Autodesk Inventor part; units mm, degrees
ref_plane "CP_XY" through (0, 0, 0) normal (0, 1, 0) x (1, 0, 0)
ref_plane "CP_YZ" through (0, 0, 0) normal (1, 0, 0) x (0, 0, -1)
ref_plane "CP_ZX" through (0, 0, 0) normal (0, 0, -1) x (0, 1, 0)
sketch "Sketch_1" plane through (0, 0, 0) normal (1, 0, 0) x (0, 1, 0)
  line L0 (6.8, 43.4562) -> (3.8228, 41.7889)
  arc A0 (3.8228, 41.7889) -> (2.8, 40.0439) centre (4.8, 40.0439) ccw
  line L1 (2.8, 40.0439) -> (2.8, -40.0439)
  arc A1 (2.8, -40.0439) -> (3.8228, -41.7889) centre (4.8, -40.0439) ccw
  line L2 (3.8228, -41.7889) -> (5.3114, -42.6226)
  arc A2 (5.3114, -42.6226) -> (6.8, -41.7501) centre (5.8, -41.7501) ccw
  line L3 (6.8, -41.7501) -> (6.8, 43.4562)
extrude "Extrusion1" add sketch "Sketch_1" along normal mid plane 22.5
sketch "Sketch_4" plane through (0, 0, 0) normal (1, 0, 0) x (0, 1, 0)
  line L0 (6.78, 48.4) -> (-1, 48.4)
  line L1 (-1, 48.4) -> (-1, -48.4)
  line L2 (-1, -48.4) -> (6.78, -48.4)
  line L3 (6.78, -48.4) -> (7.1588, -48.2985)
  arc A0 (7.1588, -48.2985) -> (7.9, -47.3326) centre (6.9, -47.3326) ccw
  line L4 (7.9, -47.3326) -> (7.9, -45.0762)
  arc A1 (7.9, -45.0762) -> (7.3886, -44.2037) centre (6.9, -45.0762) ccw
  line L5 (7.3886, -44.2037) -> (5.4, -43.09)
  line L6 (5.4, -43.09) -> (5.4, 43.09)
  line L7 (5.4, 43.09) -> (7.3886, 44.2037)
  arc A2 (7.3886, 44.2037) -> (7.9, 45.0762) centre (6.9, 45.0762) ccw
  line L8 (7.9, 45.0762) -> (7.9, 47.3326)
  arc A3 (7.9, 47.3326) -> (7.1588, 48.2985) centre (6.9, 47.3326) ccw
  line L9 (7.1588, 48.2985) -> (6.78, 48.4)
extrude "Extrusion2" cut sketch "Sketch_4" along normal mid plane 20
sketch "Sketch_10" plane through (5.5, 0, 0) normal (1, 0, 0) x (0, 0, -1)
  line L0 (-43.5, 6.7302) -> (-42.755, 5.4)
  line L1 (-42.755, 5.4) -> (-42.2975, 5.4)
  line L2 (-42.2975, 5.4) -> (-41.9848, 7.1736)
  arc A0 (-40.0152, 7.1736) -> (-41.9848, 7.1736) centre (-41, 7) ccw
  line L3 (-40.0152, 7.1736) -> (-39.7025, 5.4)
  line L4 (-39.7025, 5.4) -> (-37.8117, 5.4)
  line L5 (-37.8117, 5.4) -> (-39.255, 7.9772)
  arc A1 (-39.255, 7.9772) -> (-42.7116, 8.0346) centre (-41, 7) ccw
  line L6 (-42.7116, 8.0346) -> (-43.5, 6.7302)
extrude "Extrusion3" add sketch "Sketch_10" against normal blind 1.4
sketch "Sketch_2" plane through (-5.5, 0, 0) normal (1, 0, 0) x (0, 0, -1)
  line L0 (-43.5, 6.7302) -> (-42.755, 5.4)
  line L1 (-42.755, 5.4) -> (-42.2975, 5.4)
  line L2 (-42.2975, 5.4) -> (-41.9848, 7.1736)
  arc A0 (-40.0152, 7.1736) -> (-41.9848, 7.1736) centre (-41, 7) ccw
  line L3 (-40.0152, 7.1736) -> (-39.7025, 5.4)
  line L4 (-39.7025, 5.4) -> (-37.8117, 5.4)
  line L5 (-37.8117, 5.4) -> (-39.255, 7.9772)
  arc A1 (-39.255, 7.9772) -> (-42.7116, 8.0346) centre (-41, 7) ccw
  line L6 (-42.7116, 8.0346) -> (-43.5, 6.7302)
extrude "Extrusion4" add sketch "Sketch_2" along normal blind 1.4
sketch "Sketch_3" plane through (0, 0, 0) normal (1, 0, 0) x (0, 1, 0)
  line L0 (7.3, 45) -> (2.8, 45)
  line L1 (2.8, 45) -> (2.8, 41.2161)
  line L2 (2.8, 41.2161) -> (6.7545, 43.4307)
  arc A0 (6.8522, 43.4562) -> (6.7545, 43.4307) centre (6.8522, 43.2562) ccw
  line L3 (6.8522, 43.4562) -> (7.3, 43.4562)
  line L4 (7.3, 43.4562) -> (7.3, 45)
extrude "Extrusion5" cut sketch "Sketch_3" along normal mid plane 24
sketch "Sketch_5" plane through (0, 6.8, 0) normal (0, 1, 0) x (1, 0, 0)
  line L0 (-4.1, -38.44) -> (-4.1, -47)
  line L1 (-4.1, -47) -> (4.1, -47)
  line L2 (4.1, -47) -> (4.1, -38.44)
  line L3 (4.1, -38.44) -> (1.9, -38.44)
  line L4 (1.9, -38.44) -> (1.9, -45)
  line L5 (1.9, -45) -> (-1.9, -45)
  line L6 (-1.9, -45) -> (-1.9, -38.44)
  line L7 (-1.9, -38.44) -> (-4.1, -38.44)
extrude "Extrusion6" cut sketch "Sketch_5" against normal blind 1.5
sketch "Sketch_6" plane through (5.5, 0, 0) normal (1, 0, 0) x (0, 0, -1)
  line L0 (-42.2975, 5.4) -> (-39.7025, 5.4)
  line L1 (-39.7025, 5.4) -> (-40.0152, 7.1736)
  arc A0 (-40.0152, 7.1736) -> (-41.9848, 7.1736) centre (-41, 7) ccw
  line L2 (-41.9848, 7.1736) -> (-42.2975, 5.4)
extrude "Extrusion7" cut sketch "Sketch_6" against normal blind 1.5
sketch "Sketch_7" plane through (-5.5, 0, 0) normal (1, 0, 0) x (0, 0, -1)
  line L0 (-42.2975, 5.4) -> (-39.7025, 5.4)
  line L1 (-39.7025, 5.4) -> (-40.0152, 7.1736)
  arc A0 (-40.0152, 7.1736) -> (-41.9848, 7.1736) centre (-41, 7) ccw
  line L2 (-41.9848, 7.1736) -> (-42.2975, 5.4)
extrude "Extrusion8" cut sketch "Sketch_7" along normal blind 1.5
sketch "Sketch_8" plane through (0, 6.8, 0) normal (0, 1, 0) x (1, 0, 0)
  line L0 (-9.1, 46) -> (-9.1, 38.25)
  arc A0 (-9.1, 38.25) -> (-8.5, 37.65) centre (-8.5, 38.25) ccw
  line L1 (-8.5, 37.65) -> (-7.331, 37.65)
  arc A1 (-7.331, 37.65) -> (-7.0913, 37.829) centre (-7.331, 37.9) ccw
  line L2 (-7.0913, 37.829) -> (-6.7103, 39.1152)
  arc A2 (-6.7103, 39.1152) -> (-6.7, 39.1862) centre (-6.95, 39.1862) ccw
  line L3 (-6.7, 39.1862) -> (-6.7, 44)
  line L4 (-6.7, 44) -> (6.7, 44)
  line L5 (6.7, 44) -> (6.7, 39.1862)
  arc A3 (6.7, 39.1862) -> (6.7103, 39.1152) centre (6.95, 39.1862) ccw
  line L6 (6.7103, 39.1152) -> (7.0913, 37.829)
  arc A4 (7.0913, 37.829) -> (7.331, 37.65) centre (7.331, 37.9) ccw
  line L7 (7.331, 37.65) -> (8.5, 37.65)
  arc A5 (8.5, 37.65) -> (9.1, 38.25) centre (8.5, 38.25) ccw
  line L8 (9.1, 38.25) -> (9.1, 46)
  line L9 (9.1, 46) -> (-9.1, 46)
extrude "Extrusion9" cut sketch "Sketch_8" against normal blind 1.5
sketch "Sketch_11" plane through (0, 6.8, 0) normal (0, 1, 0) x (1, 0, 0)
  line L0 (-6.95, 28.75) -> (6.95, 28.75)
  line L1 (6.95, 28.75) -> (6.95, 37.05)
  line L2 (6.95, 37.05) -> (-6.95, 37.05)
  line L3 (-6.95, 37.05) -> (-6.95, 28.75)
extrude "Extrusion10" cut sketch "Sketch_11" against normal blind 0.5
sketch "Sketch_13" plane through (0, 6.8, 0) normal (0, 1, 0) x (1, 0, 0)
  circle A0 centre (-5, 32.9) radius 0.6
extrude "Extrusion11" cut sketch "Sketch_13" against normal blind 1.5
sketch "Sketch_14" plane through (0, 6.8, 0) normal (0, 1, 0) x (1, 0, 0)
  circle A0 centre (5, 32.9) radius 0.6
extrude "Extrusion12" cut sketch "Sketch_14" against normal blind 1.5
ref_plane "CP_XY" through (0, 0, 0) normal (0, 1, 0) x (1, 0, 0)
ref_plane "CP_YZ" through (0, 0, 0) normal (1, 0, 0) x (0, 0, -1)
ref_plane "CP_ZX" through (0, 0, 0) normal (0, 0, -1) x (0, 1, 0)
ref_plane "mitFront_XY" through (0, 7, 41) normal (1, 0, 0) x (0, 0, -1)
ref_plane "mitFront_YZ" through (0, 7, 41) normal (0, 0, -1) x (0, 1, 0)
ref_plane "mitFront_ZX" through (0, 7, 41) normal (0, 1, 0) x (1, 0, 0)
ref_plane "mitMark_XY" through (0, 6.3, -32.9) normal (0, -1, 0) x (1, 0, 0)
ref_plane "mitMark_YZ" through (0, 6.3, -32.9) normal (1, 0, 0) x (0, 0, 1)
ref_plane "mitMark_ZX" through (0, 6.3, -32.9) normal (0, 0, 1) x (0, -1, 0)
properties part number "CH20M22 C BK 2418670000"
The listing builds one solid part. Answer for the finished solid, in the listing's coordinates (mm). A direction names the side the tool comes from. Coordinates: 2 decimals unless noted, no trailing zeros. Write each loop counter-clockwise with the first axis right and the second up, starting at its lowest first coordinate (ties: lowest second). Pieces come first, ordered by that corner, then holes. Notation, with made-up numbers: M 39.25,-13 L 94.25,-13 A23 cw 94.25,0 Z; hole C -29,51.5 d3. An arc over 180 degrees is marked long. Put each result on its own line as item: value. Start each with the question number.
1. For a pull along X with two mould halves and no side action, classify faces 6 (the cylindrical face through (10.16, 6.318, -42.605)), 7 (the flat face through (0, 6.3, -33)), 8 (the flat face through (-11.25, 5, 1)) as pulls with the +X half, pulls with the -X half, needs draft (parallel to the pull), parting line crosses it, or undercut.
2. A cutting plane is placed at C-C on x = -0.75. Write down the section's boundary in (y, z), then the cut area to 3 significant figures.
3. Flat-ended cylindrical pins translate along their axes: P1, Ø12, axis at x = -4.5, z = 31, coming from the -Y side; P2, Ø0.9, axis at x = 8, y = 6.5, coming from the -Z side; P3, Ø3, axis at x = -5.5, z = -2.5, coming from the +Y side; P4, Ø0.7, axis at y = 7.5, z = 42, coming from the -X side. Find the tip coordinate at first contact, or state that the pin passes through.
4. A cutting plane is placed at A-A on x = 3.25. Write down the section's boundary in (y, z), then the cut area to 3 significant figures.
5. Which of the six approach directions +Z, -Z, +X, -X, +Y, -Y give full straight-line access (tool end or side, diameter ignored) to faces 1 (the cylindrical face through (5, 9, 41)), 2 (the flat face through (-6.7, 6, -41)), 3 (the flat face through (-4.1, 8, 40)), 4 (the flat face through (10, 4, 1)), 5 (the flat face through (-4.81, 6.3, 39.86))?
6. A cutting plane is placed at B-B on z = -20.5. Write down the section's boundary in (x, y), then the cut area to 3 significant figures.
7. Consider line 1 (X direction, y = 5.65, z = -32.9); line 2 (X direction, y = 5, z = 40); line 3 (Z direction, x = 5, y = 5.7). Determine where each line is inside the solid, lowest interval first. Write a range as from..to.
Resolved:
1. face 6: needs draft
1. face 7: undercut
1. face 8: pulls with the -X half
2. outline: M 5.4,-42.67 A1 ccw 6.8,-41.75 L 6.8,-37.05 L 6.3,-37.05 L 6.3,-28.75 L 6.8,-28.75 L 6.8,43.45 A0.2 ccw 6.75,43.43 L 5.4,42.67 Z
2. area: 116 mm2
3. P1: stops at y = 2.8
3. P2: stops at z = -37.65
3. P3: stops at y = 6.8
3. P4: stops at x = -5.5
4. outline: M 5.4,-42.67 A1 ccw 6.8,-41.75 L 6.8,-37.05 L 6.3,-37.05 L 6.3,-28.75 L 6.8,-28.75 L 6.8,38.44 L 5.4,38.44 Z
4. area: 109 mm2
5. face 1: +X, -X, +Y
5. face 2: -Z, +Y, -Y
5. face 3: +Z, +Y, -Y
5. face 4: +Z, -Z, -Y
5. face 5: -Y
6. outline: M -11.25,2.8 L -10,2.8 L -10,5.4 L 10,5.4 L 10,2.8 L 11.25,2.8 L 11.25,6.8 L -11.25,6.8 Z
6. area: 38.0 mm2
7. line 1: x = -11.25..-5.6, -4.4..4.4, 5.6..11.25
7. line 2: x = -11.25..-10, 10..11.25
7. line 3: z = -42.75..-33.5, -32.3..39.76, 42.24..42.84
